```python
from build123d import *

# Parameters (mm, degrees)
SKETCH1_R               = 25
BOSS_EXTRUDE1_DEPTH     = 50
SKETCH2_R               = 6
CUT_EXTRUDE1_DEPTH      = 26
CUT_EXTRUDE1_DEPTH_BACK = 60
SKETCH3_R               = 12.5
BOSS_EXTRUDE2_DEPTH     = 500


with BuildPart() as part:
    # Sketch1 → Boss-Extrude1 (new body)
    with BuildSketch(Plane(origin=(0, 0, 0), x_dir=(0, 0, -1), z_dir=(1, 0, 0))):
        Circle(SKETCH1_R)
    extrude(amount=BOSS_EXTRUDE1_DEPTH)

    # Sketch2 → Cut-Extrude1 (cut, two sides)
    with BuildSketch(Plane.XY) as cut_extrude1_sk:
        with Locations((25, 0)):
            Circle(SKETCH2_R)
    extrude(amount=CUT_EXTRUDE1_DEPTH, mode=Mode.SUBTRACT)
    extrude(cut_extrude1_sk.sketch, amount=-CUT_EXTRUDE1_DEPTH_BACK, mode=Mode.SUBTRACT)

    # Sketch3 → Boss-Extrude2 (add)
    with BuildSketch(Plane(origin=(50, 0, 0), x_dir=(0, 0, -1), z_dir=(1, 0, 0))):
        Circle(SKETCH3_R)
    extrude(amount=BOSS_EXTRUDE2_DEPTH)


solid = part.part
```
The listing builds one solid part. Answer for the finished solid, in the listing's coordinates (mm). A direction names the side the tool comes from. Give positions to 0.01 mm unless a question says otherwise; leave off trailing zeros. Loops run counter-clockwise (first coordinate to the right, second up) from the corner with the lowest first, then second, coordinate; pieces in that order, holes last. Notation, with made-up numbers: (88.25, -10.5) - (138.25, -10.5) arc R24 ccw to (138.25, 5.5) - close; hole circle Ø8 at (-34, 1). An arc over 180 degrees is marked (long way). Answer as CSV lines item,"result". Start each with the question number.
Item 1: A cutting plane is placed at B-B on z = 0. Determine the outline of the cut face in (x, y).
Item 2: Each of these flat-tipped pins is pushed along its axis until it touches: pin 1 (1 mm diameter, centred on x = 171.5, y = 4, fed in from -Z); pin 2 (12 mm diameter, centred on x = 201.5, y = -17, fed in from +Z); pin 3 (8 mm diameter, centred on x = 230, z = 13, fed in from -Y). Where does it stop, or does it pass through?
Item 3: A cutting plane is placed at C-C on x = 456. Determine the outline of the cut face in (y, z), then the cut area to 3 significant figures.
Item 4: The mould has two halves that part along X. Classify faces 1 (the face through (20.24, -3.65, 0.35)), 2 (the face through (0, 0, 0)), 3 (the face through (50, 5.9, 11.5)): +X half, -X half, draft (parallel to the pull), parting line (faces both ways), or undercut.
Item 5: A cutting plane is placed at D-D on x = 25. Determine the outline of the cut face in (y, z), then the cut area to 3 significant figures.
Item 6: For faces 4 (the face through (296.5, 3.755, -11.923)), 5 (the face through (24.65, 7.509, -23.846)), determine the directions among +Z, -Z, +X, -X, +Y, -Y from which every point of the face is accessible in a straight line to the end or side of a thin tool.
Item 7: A cutting plane is placed at A-A on y = 0. Determine the outline of the cut face in (x, z).
Item 8: Find the intervals of material crossed by line 1 (X direction, y = 0, z = 12); line 2 (Y direction, x = 25, z = 1); line 3 (Y direction, x = 25, z = -9), in increasing order. Write a range as from..to.
Found:
1,outline,"(0, -25) - (50, -25) - (50, -12.5) - (550, -12.5) - (550, 12.5) - (50, 12.5) - (50, 25) - (0, 25) - close; hole circle Ø12 at (25, 0)"
2,pin 1,"stops at z = -12"
2,pin 2,"stops at z = 5.94"
2,pin 3,"stops at y = -8.67"
3,outline,"circle Ø25 at (0, 0)"
3,area,"491 mm^2"
4,face 1,"undercut"
4,face 2,"-X half"
4,face 3,"+X half"
5,outline,"(-6, -24.27) - (-6, 24.27) arc R25 ccw to start; (6, -24.27) arc R25 ccw to (6, 24.27) - close"
5,area,"1,370 mm^2"
6,face 4,"+X"
6,face 5,"+X, -X"
7,outline,"(0, -25) - (19, -25) - (19, 25) - (0, 25) - close; (31, -25) - (50, -25) - (50, -12.5) - (550, -12.5) - (550, 12.5) - (50, 12.5) - (50, 25) - (31, 25) - close"
8,line 1,"x = 0..19, 31..550"
8,line 2,"y = -24.98..-6, 6..24.98"
8,line 3,"y = -23.32..-6, 6..23.32"
